CAD build for the part. Positions are in the model's coordinates, mm. Face numbers are marked on the shaded views. Coordinates: 2 decimals unless noted, no trailing zeros. Order: outer loops, then holes, each group sorted by start corner. A loop starts at its lowest first (then second) coordinate and runs counter-clockwise, first axis right, second up. Notation, with made-up numbers: (48, -30) - (66, -30) arc R13 ccw to (66, -25) - close; hole circle Ø7 at (-37, 66.25). An arc over 180 degrees is marked (long way). Use one line per item in the form item = value.
Autodesk Inventor part; units mm, degrees
ref_plane "YZ Plane" through (0, 0, 0) normal (1, 0, 0) x (0, 1, 0)
ref_plane "XZ Plane" through (0, 0, 0) normal (0, 1, 0) x (-1, 0, 0)
ref_plane "XY Plane" through (0, 0, 0) normal (0, 0, 1) x (1, 0, 0)
sketch "Sketch1" plane through (0, 0, 0) normal (0, 0, 1) x (1, 0, 0)
  line L0 (97.2346, 27.952) -> (-27.7654, 27.952)
  line L1 (-27.7654, 27.952) -> (-27.7654, -97.248)
  line L2 (-27.7654, -97.248) -> (97.2346, -97.248)
  line L3 (97.2346, -97.248) -> (97.2346, 27.952)
  line L4 (85.1346, 27.952) -> (85.1346, -97.248) construction
  line L5 (-15.4654, 27.952) -> (-15.4654, -97.248) construction
  line L6 (-37.3152, 15.652) -> (117.1466, 15.652) construction
  line L7 (115.2487, -84.948) -> (-56.3615, -84.948) construction
  line L8 (34.8346, -156.7023) -> (34.8346, 57.8793) construction
  line L9 (59.9846, 68.2484) -> (59.9846, -132.2245) construction
  line L10 (9.6846, 55.4717) -> (9.6846, -128.574) construction
  point P0 (0, 0)
  point P1 (-65.7997, 171.2688)
  point P2 (85.1346, -84.948)
  point P3 (85.1346, 15.652)
  point P4 (-15.4654, 15.652)
  point P5 (-15.4654, -84.948)
  point P6 (34.8346, -84.948)
  point P7 (34.8346, 15.652)
  point P8 (59.9846, 15.652)
  point P9 (9.6846, 15.652)
  point P10 (59.9846, -84.948)
  point P11 (9.6846, -84.948)
  dimension "d0" = 125
  dimension "d1" = 125.2
  dimension "d6" = 100.6
  dimension "d48" = 12.3
  dimension "d49" = 100.6
  dimension "d50" = 50.3
  dimension "d72" = 25.15
  dimension "d73" = 25.15
extrude "Extrusion1" add sketch "Sketch1" along normal blind 6
hole "Hole6" at (85.1346, -84.948, 0) at (34.8346, -84.948, 0) at (-15.4654, -84.948, 0) direction (0, 0, 1) diameter 5.1 end through all counterbore diameter 9.2 counterbore depth 3
sketch "Sketch2" plane through (0, 0, 6) normal (0, 0, 1) x (1, 0, 0)
  line L0 (86.1945, -57.9789) -> (32.1694, -57.9789) construction
  line L1 (32.1694, -57.9789) -> (32.1694, -50.1092) construction
  line L2 (32.1694, -50.1092) -> (86.1945, -50.1092) construction
  line L3 (86.1945, -50.1092) -> (86.1945, -57.9789) construction
  point P0 (0, 0)
sketch "Sketch3" plane through (0, 0, 0) normal (0, 0, -1) x (-1, 0, 0)
  point P0 (0, 0)
hole "Hole7" at (85.1346, 15.652, 0) at (34.8346, 15.652, 0) at (-15.4654, 15.652, 0) direction (0, 0, 1) diameter 7.2 end through all counterbore diameter 12.25 counterbore depth 3
sketch "Sketch5" plane through (0, 0, 0) normal (0, 0, -1) x (-1, 0, 0)
  line L0 (27.7654, -97.248) -> (-97.2346, -97.248) construction
  line L1 (-97.2346, -97.248) -> (-97.2346, 27.952) construction
  line L2 (27.7654, 27.952) -> (27.7654, -97.248) construction
  line L3 (-97.2346, 27.952) -> (27.7654, 27.952) construction
  line L4 (-97.2346, -97.248) -> (-97.2346, 27.952) construction
  line L5 (-97.2346, -34.648) -> (27.7654, -34.648) construction
  line L6 (27.7654, 27.952) -> (27.7654, -97.248) construction
  line L7 (-97.2346, -44.648) -> (27.7654, -44.648) construction
  line L8 (-97.2346, -24.648) -> (27.7654, -24.648) construction
  line L9 (27.7654, -97.248) -> (-97.2346, -97.248) construction
  line L10 (-34.7346, -97.248) -> (-34.7346, 27.952) construction
  line L11 (-97.2346, 27.952) -> (27.7654, 27.952) construction
  point P0 (0, 0)
  point P1 (-34.7346, -44.648)
  point P2 (-34.7346, -24.648)
  dimension "d81" = 10
  dimension "d82" = 10
hole "Hole8" at (34.7346, -44.648, 0) at (34.7346, -24.648, 0) direction (0, 0, 1) diameter 5.1 end through all counterbore diameter 9.2 counterbore depth 3
hole "Hole9" at (59.9846, 15.652, 0) at (9.6846, 15.652, 0) at (59.9846, -84.948, 0) at (9.6846, -84.948, 0) direction (0, 0, 1) diameter 4.2 end through all
equation "\"d72\" = 0.5 * d50"
equation "\"d73\" = 0.5 * d50"
properties part number "X axis carriage small_3DPrint"
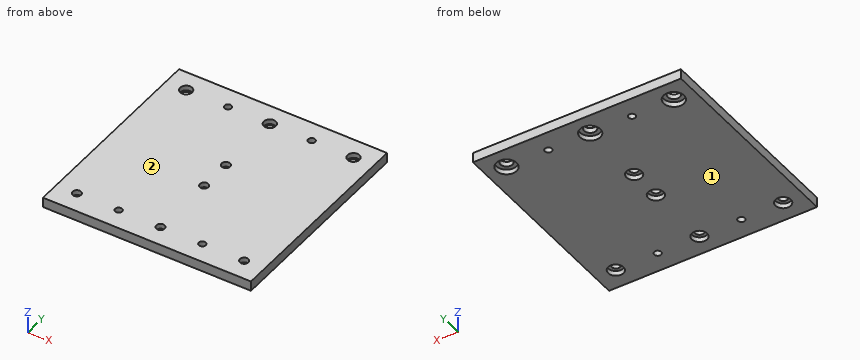
Item 1: Two-plate mould, pull along Z, no slides. Class the marked faces 1 and 2: +Z half, -Z half, draft (parallel to the pull), parting line (faces both ways), or undercut.
Derived:
face_1 = -Z half
face_2 = +Z half
Item 2: Drill centre lines: line 1 (Y direction, x = 35, z = 1.3); line 2 (X direction, y = 20.5, z = 2.3); line 3 (Y direction, x = 59, z = 1.1). Where is each one in solid material? Low to high. Write a range as [from, to].
Derived:
line_1 = [-97.25, -89.55], [-80.35, -49.24], [-40.06, -29.24], [-20.06, 9.53], [21.77, 27.95]
line_2 = [-27.77, -19.21], [-11.72, 31.09], [38.58, 81.39], [88.88, 97.23]
line_3 = [-97.25, -86.8], [-83.09, 13.8], [17.51, 27.95]
Item 3: Cut at B-B, the plane y = -24. Write the cut outline in (x, z).
Derived:
outline = (-27.77, 0) - (30.18, 0) - (30.18, 3) - (32.27, 3) - (32.27, 6) - (-27.77, 6) - close; (37.2, 3) - (39.29, 3) - (39.29, 0) - (97.23, 0) - (97.23, 6) - (37.2, 6) - close
Item 4: Drop flat-ended pins along their axis: pin 1 (4.5 mm diameter, centred on x = -18, y = -86.5, fed in from -Z); pin 2 (6.5 mm diameter, centred on x = -15.47, y = 15.65, fed in from +Z); pin 3 (8.5 mm diameter, centred on x = -15.47, y = -84.95, fed in from -Z). Give the stop position or say it passes through.
Derived:
pin_1 = 0
pin_2 = through
pin_3 = 3
Item 5: Cut at A-A, the plane z = 4.35. State how many separate pieces and enclosed holes the cut face has, plus the area to 3 significant figures.
Derived:
separate_pieces = 1
enclosed_holes = 12
area = 15,400 mm²
